Read the model definition and answer for the solid it produces. Units are mm, in the model's axes. A direction names the side the tool comes from. Give positions to 0.01 mm unless a question says otherwise; leave off trailing zeros. Order: outer loops, then holes, each group sorted by start corner. A loop starts at its lowest first (then second) coordinate and runs counter-clockwise, first axis right, second up. Notation, with made-up numbers: (62.5, 27) - (118.5, 27) arc R11 cw to (118.5, 42) - close; hole circle Ø5 at (88, 43.5). An arc over 180 degrees is marked (long way). Use a Markdown table: item, result. Add a question column.
1. Flat-ended cylindrical pins translate along their axes: P1, Ø15, axis at y = 1.5, z = -24.5, coming from the -X side; P2, Ø8, axis at x = -30.5, y = 9.5, coming from the +Z side; P3, Ø16.5, axis at x = -32, z = -60.5, coming from the -Y side. Find the tip coordinate at first contact, or state that the pin passes through.
2. A cutting plane is placed at C-C on y = -28. State how many separate pieces and enclosed holes the cut face has, and give its area (3 significant figures).
3. For a pull along Z with two mould halves and no side action, classify faces 4 (the flat face through (-42, 6, -50)), 5 (the cylindrical face through (-28.59, -26.69, 18.74)), 6 (the flat face through (-34, 45.209, -58)) as released by +Z, released by -Z, zero draft, split by the parting line, or undercut.
4. A cutting plane is placed at D-D on y = 36. Determine the outline of the cut face in (x, z), and give its area (3 significant figures).
5. A cutting plane is placed at A-A on z = -57. Determine the outline of the cut face in (x, y).
6. Which of the six approach directions +Z, -Z, +X, -X, +Y, -Y give full straight-line access (tool end or side, diameter ignored) to faces 1 (the flat face through (0, -28, 22)), 2 (the flat face through (-40, -6, -27)), 3 (the flat face through (-22.509, 5, -43))?
7. A cutting plane is placed at B-B on x = -32.5. Determine the outline of the cut face in (y, z).
8. Consider L1, parallel to Y at x = -37.5, z = -51; L2, parallel to Z at x = -33, y = -24; L3, parallel to Z at x = -17.5, y = -19.5. Determine where each line is inside the solid, lowest interval first.
```python
from build123d import *

# Parameters (mm, degrees)
F2_R      = 40
F2_R_2    = 23
F4_DEPTH  = 34
F8_DEPTH  = 25
F10_DEPTH = 34
F11_DEPTH = 133
F13_DEPTH = 262


with BuildPart() as f4:
    # F2 (on face) → F4 (new body)
    with BuildSketch(Plane(origin=(0, 0, 0), x_dir=(-1, 0, 0), z_dir=(0, 0.9135454576, 0.4067366431))):
        Circle(F2_R)
        Circle(F2_R_2, mode=Mode.SUBTRACT)
    extrude(amount=-F4_DEPTH)



with BuildPart() as f8:
    # F7 (on offset) → F8 (new body)
    with BuildSketch(Plane.YZ.offset(-46)):
        Polygon((45.2089201632, -50), (22.2614342654, -50), (28.9398645451, -65), (45.2089201632, -65), align=None)
        Polygon((22.2614342654, -50), (-14.9561992038, -50), (-14.7910798368, -50.3708641703), (-8.2777689242, -65), (28.9398645451, -65), align=None)
        Polygon((-14.7910798368, -50.3708641703), (-14.7910798368, -65), (-8.2777689242, -65), align=None)
        Polygon((-14.9561992038, -50), (-34.7910798368, -50), (-34.7910798368, -65), (-14.7910798368, -65), (-14.7910798368, -50.3708641703), align=None)
    extrude(amount=F8_DEPTH)


with BuildPart() as f4_1:
    add(f4.part)

    add(f8.part)  # F10 merges F8
    # F9 (on face) → F10 (join, through all)
    with BuildSketch(Plane(origin=(0, 0, 0), x_dir=(-1, 0, 0), z_dir=(0, 0.9135454576, 0.4067366431))):
        with BuildLine():
            Line((40, -125.3134310246), (40, 0))
            ThreePointArc((40, 0), (35.3578901582, -18.7034650149), (22.5090198219, -33.0657530786))
            Line((22.5090198219, -33.0657530786), (22.5090198219, -125.3134310246))
            Line((22.5090198219, -125.3134310246), (40, -125.3134310246))
        make_face()
    extrude(amount=-F10_DEPTH)

    # F11 (cut): a face of the model
    f11_faces = [f4_1.faces().sort_by_distance(p)[0] for p in [
        (-22.5090198219, 22.1875323244, -93.3383186081),
    ]]
    extrude(f11_faces, amount=-F11_DEPTH, mode=Mode.SUBTRACT)

    # F12 (on face) → F13 (cut)
    with BuildSketch(Plane(origin=(0, 0, 0), x_dir=(-1, 0, 0), z_dir=(0, 0.9135454576, 0.4067366431))):
        with BuildLine():
            Line((0, 23), (0, 40))
            ThreePointArc((0, 40), (-28.2842712475, 28.2842712475), (-40, 0))
            Line((-40, 0), (-23, 0))
            ThreePointArc((-23, 0), (-16.2634559673, 16.2634559673), (0, 23))
        make_face()
    extrude(amount=-F13_DEPTH, mode=Mode.SUBTRACT)


solid = f4_1.part
```
Output values:
| question | item | result |
|---|---|---|
| 1 | P1 | x = -40 |
| 1 | P2 | z = -12.35 |
| 1 | P3 | y = -34.79 |
| 2 | separate pieces | 3 |
| 2 | enclosed holes | 0 |
| 2 | area | 1,580 mm² |
| 3 | face 4 | undercut |
| 3 | face 5 | released by +Z |
| 3 | face 6 | zero draft |
| 4 | outline | (-46, -65) - (-21, -65) - (-21, -50) - (-46, -50) - close |
| 4 | area | 375 mm² |
| 5 | outline | (-46, -34.79) - (-21, -34.79) - (-21, 45.21) - (-46, 45.21) - close |
| 6 | face 1 | +Z, +X, +Y, -Y |
| 6 | face 2 | +Z, -X, +Y, -Y |
| 6 | face 3 | +Y |
| 7 | outline | (-40.55, 7.47) - (-14.96, -50) - (-34.79, -50) - (-34.79, -65) - (45.21, -65) - (45.21, -50) - (22.26, -50) - (-9.48, 21.3) - close |
| 8 | L1 | -34.79 to 45.21 |
| 8 | L2 | -65 to -50, -29.69 to 14.06 |
| 8 | L3 | -39.79 to -25.02, 7.66 to 30.69 |
